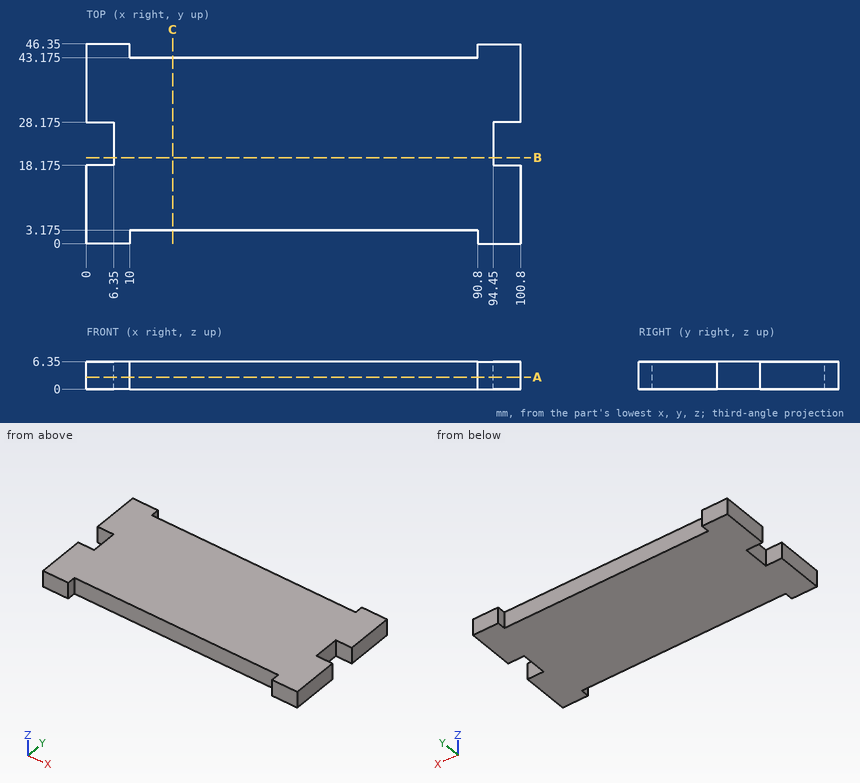
Design review of the part shown in the three views and the two pictorial views. Dimensions are in mm from the part's minimum x, y and z. Give positions to 0.01 mm unless a question says otherwise; leave off trailing zeros. Loops run counter-clockwise (first coordinate to the right, second up) from the corner with the lowest first, then second, coordinate; pieces in that order, holes last. Notation, with made-up numbers: (28, -25) - (75, -25) arc R8 cw to (75, -13) - close; hole circle Ø5 at (23.5, -25). An arc over 180 degrees is marked (long way). Use CSV: the item, a comma, the result in double quotes. Start each with the question number.
1. Wall thickness on L1, parallel to X at y = 3, z = 3.25; L2, parallel to Y at x = 61.5, z = 1.5 (3 decimals); L3, parallel to X at y = 25, z = 0.75: over which ranges is each line inside the solid? List them lowest first.
2. Add section C-C (x = 20). State the section outline as (y, z) points (3 decimals).
3. Add section B-B (y = 20). State the section outline as (x, z) points, plus the area to 3 significant figures.
4. Insertion check: P1, Ø2, axis at y = 19.5, z = 2.5, coming from the +X side. The pin has a flat end and moves straight along its axis. Give the tip position at first contact, or say it passes through.
5. Add section A-A (z = 2.75). State the section outline as (x, y) points (3 decimals).
Results found:
1,L1,"x = 0 to 10, 90.8 to 100.8"
1,L2,"y = 3.175 to 43.175"
1,L3,"x = 6.35 to 94.45"
2,outline,"(3.175, 0) - (43.175, 0) - (43.175, 6.35) - (3.175, 6.35) - close"
3,outline,"(6.35, 0) - (94.45, 0) - (94.45, 6.35) - (6.35, 6.35) - close"
3,area,"559 mm²"
4,P1,"stops at x = 94.45"
5,outline,"(0, 0) - (10, 0) - (10, 3.175) - (90.8, 3.175) - (90.8, 0) - (100.8, 0) - (100.8, 18.175) - (94.45, 18.175) - (94.45, 28.175) - (100.8, 28.175) - (100.8, 46.35) - (90.8, 46.35) - (90.8, 43.175) - (10, 43.175) - (10, 46.35) - (0, 46.35) - (0, 28.175) - (6.35, 28.175) - (6.35, 18.175) - (0, 18.175) - close"
